```python
from build123d import *

# Parameters (mm, degrees)
SKETCH1_R               = 19.05
BOSS_EXTRUDE1_DEPTH     = 6.35
SKETCH3_R               = 6.985
CUT_EXTRUDE2_DEPTH      = 6.35
CUT_EXTRUDE1_DEPTH      = 6.35
CUT_EXTRUDE3_DEPTH      = 125.954641054
CUT_EXTRUDE3_DEPTH_BACK = 125.954641054
SKETCH4_R               = 2.159
SKETCH6_R               = 6.985
BOSS_EXTRUDE2_DEPTH     = 6.35


with BuildPart() as part:
    # Sketch1 → Boss-Extrude1 (new body)
    with BuildSketch(Plane(origin=(0, 0, 0), x_dir=(0, 0, -1), z_dir=(1, 0, 0))):
        with BuildLine():
            Line((25.4, 62.611), (-25.4, 62.611))
            ThreePointArc((-25.4, 62.611), (-43.71389723, 59.350669702), (-59.777434529, 49.970298982))
            Line((-59.777434529, 49.970298982), (-101.281034529, 14.478))
            ThreePointArc((-101.281034529, 14.478), (-80.929937509, 17.302618411), (-69.85, 0))
            ThreePointArc((-69.85, 0), (-80.929937509, -17.302618411), (-101.281034529, -14.478))
            Line((-101.281034529, -14.478), (-59.777434529, -49.970298982))
            ThreePointArc((-59.777434529, -49.970298982), (-43.71389723, -59.350669702), (-25.4, -62.611))
            Line((-25.4, -62.611), (25.4, -62.611))
            ThreePointArc((25.4, -62.611), (43.699078076, -59.34404997), (59.737214243, -49.946847768))
            Line((59.737214243, -49.946847768), (101.269374674, -14.487973703))
            ThreePointArc((101.269374674, -14.487973703), (69.85, -7.706e-06), (101.269379322, 14.48794821))
            Line((101.269379322, 14.48794821), (59.737230268, 49.9468356))
            ThreePointArc((59.737230268, 49.9468356), (43.699087699, 59.344046737), (25.4, 62.611))
        make_face()
        with Locations((88.9, -1.0762e-05)):
            Circle(SKETCH1_R)
        with Locations((-88.9, 0)):
            Circle(SKETCH1_R)
    extrude(amount=BOSS_EXTRUDE1_DEPTH)

    # Sketch3 → Cut-Extrude2 (cut)
    with BuildSketch(Plane(origin=(6.35, 0, 0), x_dir=(0, 0, -1), z_dir=(1, 0, 0))):
        with Locations((-88.9, 0)):
            Circle(SKETCH3_R)
        with Locations((88.9, -1.0762e-05)):
            Circle(SKETCH3_R)
    extrude(amount=-CUT_EXTRUDE2_DEPTH, mode=Mode.SUBTRACT)

    # Sketch2 → Cut-Extrude1 (cut)
    with BuildSketch(Plane(origin=(6.35, 0, 0), x_dir=(0, 0, -1), z_dir=(1, 0, 0))):
        with BuildLine():
            Line((-25.4, 47.371), (25.4, 47.371))
            ThreePointArc((25.4, 47.371), (72.771, 0), (25.4, -47.371))
            Line((25.4, -47.371), (-25.4, -47.371))
            ThreePointArc((-25.4, -47.371), (-72.771, 0), (-25.4, 47.371))
        make_face()
    extrude(amount=-CUT_EXTRUDE1_DEPTH, mode=Mode.SUBTRACT)

    # Sketch4 → Cut-Extrude3 (cut, two sides: drawn at the far end of the back side and taken through both)
    with BuildSketch(Plane(origin=(6.35, 0, 0), x_dir=(0, 0, -1), z_dir=(1, 0, 0)).offset(-CUT_EXTRUDE3_DEPTH_BACK)):
        with BuildLine():
            ThreePointArc((-73.940141084, 27.832575617), (-76.984164998, 28.070231704), (-77.221821084, 25.02620779))
            Line((-77.221821084, 25.02620779), (-73.940141084, 27.832575617))
        make_face()
        with BuildLine():
            Line((-73.940141084, 27.832575617), (-77.221821084, 25.02620779))
            ThreePointArc((-77.221821084, 25.02620779), (-74.833081546, 24.404070178), (-73.421981084, 26.429391704))
            ThreePointArc((-73.421981084, 26.429391704), (-73.555659559, 27.177291242), (-73.940141084, 27.832575617))
        make_face()
        with Locations((-54.833341451, 44.171983407)):
            Circle(SKETCH4_R)
        with Locations((-30.48, 54.706186836)):
            Circle(SKETCH4_R)
        with Locations((0, 54.991)):
            Circle(SKETCH4_R)
        with Locations((30.478659799, 54.70517335)):
            Circle(SKETCH4_R)
        with Locations((54.789478539, 44.151652011)):
            Circle(SKETCH4_R)
        with Locations((75.555553066, 26.422208316)):
            Circle(SKETCH4_R)
        with Locations((92.827553066, 14.992208316)):
            Circle(SKETCH4_R)
        with Locations((92.827553066, -14.992208316)):
            Circle(SKETCH4_R)
        with Locations((75.555553066, -26.422208316)):
            Circle(SKETCH4_R)
        with Locations((54.789478539, -44.151652011)):
            Circle(SKETCH4_R)
        with Locations((30.478659799, -54.70517335)):
            Circle(SKETCH4_R)
        with Locations((0, -54.991)):
            Circle(SKETCH4_R)
        with Locations((-30.48, -54.706186836)):
            Circle(SKETCH4_R)
        with Locations((-54.833341451, -44.171983407)):
            Circle(SKETCH4_R)
        with Locations((-75.580981084, -26.429391704)):
            Circle(SKETCH4_R)
        with Locations((-92.852981084, 14.999391704)):
            Circle(SKETCH4_R)
        with Locations((-92.852981084, -14.999391704)):
            Circle(SKETCH4_R)
    extrude(amount=CUT_EXTRUDE3_DEPTH + CUT_EXTRUDE3_DEPTH_BACK, mode=Mode.SUBTRACT)

    # Sketch6 → Boss-Extrude2 (add)
    with BuildSketch(Plane(origin=(6.35, 0, 0), x_dir=(0, 0, -1), z_dir=(1, 0, 0))):
        with BuildLine():
            ThreePointArc((-71.961883, 8.717952311), (-78.500282105, 15.960838565), (-87.767121516, 19.016284767))
            ThreePointArc((-87.767121516, 19.016284767), (-88.915797503, 18.427684462), (-88.956054378, 17.137612284))
            ThreePointArc((-88.956054378, 17.137612284), (-91.72021134, 10.701152796), (-97.297574405, 14.939265075))
            ThreePointArc((-97.297574405, 14.939265075), (-97.968420164, 16.041931303), (-99.257990941, 15.987949327))
            ThreePointArc((-99.257990941, 15.987949327), (-107.95, 0), (-99.257990941, -15.987949327))
            ThreePointArc((-99.257990941, -15.987949327), (-97.968420164, -16.041931303), (-97.297574405, -14.939265075))
            ThreePointArc((-97.297574405, -14.939265075), (-91.72021134, -10.701152796), (-88.956054378, -17.137612284))
            ThreePointArc((-88.956054378, -17.137612284), (-88.915797503, -18.427684462), (-87.767121516, -19.016284767))
            ThreePointArc((-87.767121516, -19.016284767), (-78.500282105, -15.960838565), (-71.961883, -8.717952311))
            ThreePointArc((-71.961883, -8.717952311), (-72.771, 0), (-71.961883, 8.717952311))
        make_face()
        with Locations((-88.9, 0)):
            Circle(SKETCH6_R, mode=Mode.SUBTRACT)
    boss_extrude2 = extrude(amount=BOSS_EXTRUDE2_DEPTH)

    # Mirror1: Boss-Extrude2 across plane
    add(boss_extrude2.mirror(Plane.XY))


solid = part.part
```
Read the model definition and answer for the solid it produces. Units are mm, in the model's axes. A direction names the side the tool comes from. Coordinates: 2 decimals unless noted, no trailing zeros. Write each loop counter-clockwise with the first axis right and the second up, starting at its lowest first coordinate (ties: lowest second). Pieces come first, ordered by that corner, then holes. Notation, with made-up numbers: (34.5, -8.75) -> (64.5, -8.75) arc R7 cw to (64.5, -3.75) -> close; hole circle Ø8 at (24, 53). An arc over 180 degrees is marked (long way). Answer as a JSON object with one key per item and string values.
Q1. The part is cut by section A-A on z = 0. Give the vertices of the cut face in (x, y), then the cut area to 3 significant figures.
The answers:
{"outline": "(0, -62.61) -> (6.35, -62.61) -> (6.35, -57.15) -> (0, -57.15) -> close; (0, -52.83) -> (6.35, -52.83) -> (6.35, -47.37) -> (0, -47.37) -> close; (0, 47.37) -> (6.35, 47.37) -> (6.35, 52.83) -> (0, 52.83) -> close; (0, 57.15) -> (6.35, 57.15) -> (6.35, 62.61) -> (0, 62.61) -> close", "area": "139 mm2"}
Q2. Determine the mould class of faces 4 (the cylindrical face through (9.481, 15.885, -78.385)), 5 (the cylindrical face through (9.48, 10.73, -91.61)), 6 (the cylindrical face through (3.131, -59.434, -43.453)), 7 (the cylindrical face through (3.13, -0.23, -107.95)) for opening direction Y: pulls with the +Y half, pulls with the -Y half, needs draft (parallel to the pull), parting line crosses it, or undercut.
The answers:
{"face 4": "pulls with the +Y half", "face 5": "undercut", "face 6": "pulls with the -Y half", "face 7": "parting line crosses it"}
Q3. The part is cut by section D-D on z = 30.48. Give the vertices of the cut face in (x, y), then the cut area to 3 significant figures.
The answers:
{"outline": "(0, -62.37) -> (6.35, -62.37) -> (6.35, -56.87) -> (0, -56.87) -> close; (0, -52.55) -> (6.35, -52.55) -> (6.35, -47.1) -> (0, -47.1) -> close; (0, 47.1) -> (6.35, 47.1) -> (6.35, 52.55) -> (0, 52.55) -> close; (0, 56.87) -> (6.35, 56.87) -> (6.35, 62.37) -> (0, 62.37) -> close", "area": "139 mm2"}
Q4. The part is cut by section B-B on x = 10.75. Give the vertices of the cut face in (y, z) (3 decimals), then the cut area to 3 significant figures.
The answers:
{"outline": "(-19.016, -87.767) arc R1.27 ccw to (-17.138, -88.956) arc R4.445 cw (long way) to (-14.939, -97.298) arc R1.27 ccw to (-15.988, -99.258) arc R19.05 ccw to (15.988, -99.258) arc R1.27 ccw to (14.939, -97.298) arc R4.445 cw (long way) to (17.138, -88.956) arc R1.27 ccw to (19.016, -87.767) arc R19.05 ccw to (8.718, -71.962) arc R47.371 cw to (-8.718, -71.962) arc R19.05 ccw to start; (-19.016, 87.767) arc R19.05 ccw to (-8.718, 71.962) arc R47.371 cw to (8.718, 71.962) arc R19.05 ccw to (19.016, 87.767) arc R1.27 ccw to (17.138, 88.956) arc R4.445 cw (long way) to (14.939, 97.298) arc R1.27 ccw to (15.988, 99.258) arc R19.05 ccw to (-15.988, 99.258) arc R1.27 ccw to (-14.939, 97.298) arc R4.445 cw (long way) to (-17.138, 88.956) arc R1.27 ccw to start; hole circle Ø13.97 at (0, -88.9); hole circle Ø13.97 at (0, 88.9)", "area": "1,660 mm2"}
Q5. The part is cut by section C-C on z = -40.5. Give the vertices of the cut face in (x, y), then the cut area to 3 significant figures.
The answers:
{"outline": "(0, -60.41) -> (6.35, -60.41) -> (6.35, -44.9) -> (0, -44.9) -> close; (0, 44.9) -> (6.35, 44.9) -> (6.35, 60.41) -> (0, 60.41) -> close", "area": "197 mm2"}
Q6. A tool of negligible diameter and unlimited length cuts with its end or side. For faces 1 (the flat face through (3, 47.371, 0)), 2 (the cylindrical face through (9.481, 15.885, 78.385)), 3 (the cylindrical face through (3.131, 59.253, -43.944)), from which of +Z, -Z, +X, -X, +Y, -Y can it reach the whole face along a straight path? Write none if from no direction.
The answers:
{"face 1": "+X, -X", "face 2": "+X, +Y", "face 3": "-Z, +X, -X, +Y"}
Q7. Flat-ended cylindrical pins translate along their axes: pin 1 Ø5 at (x, y) = (8, -50) entering from +Z; pin 2 Ø4 at (x, y) = (6, -45.5) entering from +Z; pin 3 Ø16 at (y, z) = (49, -41.5) entering from +X. Find the tip coordinate at first contact, or state that the pin passes through.
The answers:
{"pin 1": "stops at z = 61.94", "pin 2": "stops at z = 67.34", "pin 3": "stops at x = 6.35"}
Q8. Consider line 1 (Y direction, x = 2.25, z = -8); line 2 (Y direction, x = 0.75, z = 74.5); line 3 (Z direction, x = 1.75, y = -54). Determine where each line is inside the solid, lowest interval first. Write a range as [from, to].
The answers:
{"line 1": "y = [-62.61, -47.37], [47.37, 62.61]", "line 2": "y = [-37.38, -28.3], [-24.56, 24.56], [28.3, 37.38]", "line 3": "z = [-54.32, -32.52], [-28.44, -1.92], [1.92, 28.44], [32.52, 54.38]"}
